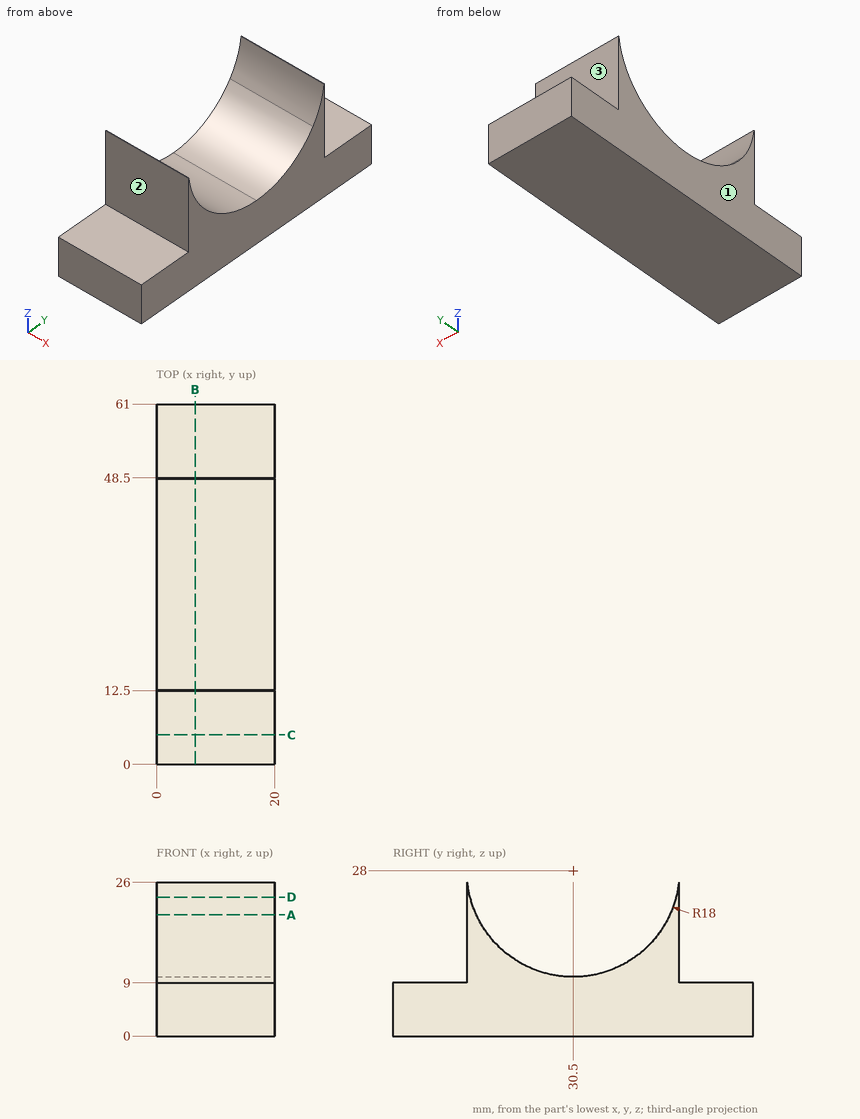
Design review of the part shown in the three views and the two pictorial views. Dimensions are in mm from the part's minimum x, y and z. A direction names the side the tool comes from. Round coordinates to 2 decimals unless told otherwise and drop trailing zeros. Loops run counter-clockwise (first coordinate to the right, second up) from the corner with the lowest first, then second, coordinate; pieces in that order, holes last.
Q1. Add section D-D on z = 23.5. Write out the cut boundary in (x, y).
Result sheet:
outline: (0, 12.5) - (20, 12.5) - (20, 13.07) - (0, 13.07) - close; (0, 47.93) - (20, 47.93) - (20, 48.5) - (0, 48.5) - close
Q2. Add section C-C on y = 5. Write out the cut boundary in (x, z).
Result sheet:
outline: (0, 0) - (20, 0) - (20, 9) - (0, 9) - close
Q3. Add section A-A on z = 20.5. Write out the cut boundary in (x, y).
Result sheet:
outline: (0, 12.5) - (20, 12.5) - (20, 14.14) - (0, 14.14) - close; (0, 46.86) - (20, 46.86) - (20, 48.5) - (0, 48.5) - close
Q4. To check wall thickness, follow line 1 along Z through (x, y) = (2.25, 58); line 2 along Z through (x, y) = (1, 30.5); line 3 along Y through (x, z) = (3.5, 14). State the ranges of each line that lie inside material, in increasing order.
Result sheet:
line 1: z = 0 to 9
line 2: z = 0 to 10
line 3: y = 12.5 to 19.19, 41.81 to 48.5
Q5. Add section B-B on x = 6.5. Write out the cut boundary in (y, z).
Result sheet:
outline: (0, 0) - (61, 0) - (61, 9) - (48.5, 9) - (48.5, 26) - (48.39, 26) arc R18 cw to (12.61, 26) - (12.5, 26) - (12.5, 9) - (0, 9) - close
Q6. Insertion check: pin 1 Ø4 at (x, y) = (5, 57) entering from +Z; pin 2 Ø1.5 at (x, z) = (14.5, 22.5) entering from -Y. Each pin has a flat end and moves straight along its axis. Give the tip position at first contact, or say it passes through.
Result sheet:
pin 1: stops at z = 9
pin 2: stops at y = 12.5
Q7. Machinability: for the marked faces 1, 2 and 3, which of the approach directions +Z, -Z, +X, -X, +Y, -Y give a long, thin tool a straight path to every point of the face, cutting with its end or side? Answer none if there is none.
Result sheet:
face 1: +Z, -Z, -X, +Y, -Y
face 2: +Z, +X, -X, -Y
face 3: +Z, +X, -X, +Y
